Design review of the part built by this model. Coordinates are the model's own, in mm. Face numbers are marked on the shaded views. A direction names the side the tool comes from. Round coordinates to 2 decimals unless told otherwise and drop trailing zeros. One line per question, with ' | ' between items. Start each with the question number.
Item 1: Machinability: for the marked faces 1, 2 and 3, which of the approach directions +Z, -Z, +X, -X, +Y, -Y give a long, thin tool a straight path to every point of the face, cutting with its end or side? Answer none if there is none.
Item 2: For L1, parallel to Y at x = 0, z = 7; L2, parallel to Y at x = 24, z = 4.25; L3, parallel to Y at x = 13.5, z = 6.25, list the stretches that pass through material, from the lowest coordinate up.
Item 3: Insertion check: pin 1 Ø6 at (x, y) = (21.5, -20.5) entering from -Z; pin 2 Ø4 at (x, y) = (20.5, -15) entering from +Z; pin 3 Ø1.2 at (y, z) = (-24.5, 4) entering from -X. Each pin has a flat end and moves straight along its axis. Give the tip position at first contact, or say it passes through.
Item 4: Draft analysis for pull direction X (two halves, no side actions). For the marked faces 4, 5 and 6, state which applies: released by +X, released by -X, zero draft, split by the parting line, or undercut.
Item 5: Add section A-A, the plane z = 1.5. Give the number of separate pieces and of enclosed holes in the cut face, and give its area (3 significant figures).
```python
from build123d import *

# Parameters (mm, degrees)
SKETCH1_R           = 5
SKETCH1_R_2         = 2.55
SKETCH1_R_3         = 1
BOSS_EXTRUDE1_DEPTH = 11
SKETCH2_R           = 19.05
SKETCH2_R_2         = 5
BOSS_EXTRUDE2_DEPTH = 1.6
CUT_EXTRUDE1_DEPTH  = 3
FILLET1_R           = 0.3
CHAMFER1_SIZE       = 0.3
CUT_EXTRUDE2_DEPTH  = 6
CHAMFER2_SIZE       = 0.3
CUT_EXTRUDE3_DEPTH  = 8
SKETCH6_R           = 9
SKETCH6_R_2         = 5
CUT_EXTRUDE4_DEPTH  = 2.6
SKETCH7_R           = 11
SKETCH7_R_2         = 9
CUT_EXTRUDE5_DEPTH  = 1.6
BOSS_EXTRUDE3_START = 3
SKETCH8_R           = 17.5
SKETCH8_R_2         = 11
BOSS_EXTRUDE3_DEPTH = 3
BOSS_EXTRUDE4_START = 7
SKETCH9_R           = 17
SKETCH9_R_2         = 11
BOSS_EXTRUDE4_DEPTH = 7
CHAMFER3_SIZE       = 0.3
CHAMFER4_SIZE       = 0.5
CHAMFER5_SIZE       = 1
CHAMFER5_SIZE2      = 1.732050808


with BuildPart() as part:
    # Sketch1 → Boss-Extrude1 (new body)
    with BuildSketch(Plane.XY):
        with BuildLine():
            Line((-25.2, 28.2), (25.2, 28.2))
            ThreePointArc((25.2, 28.2), (27.321320344, 27.321320344), (28.2, 25.2))
            Line((28.2, 25.2), (28.2, -25.2))
            ThreePointArc((28.2, -25.2), (27.321320344, -27.321320344), (25.2, -28.2))
            Line((25.2, -28.2), (-25.2, -28.2))
            ThreePointArc((-25.2, -28.2), (-27.321320344, -27.321320344), (-28.2, -25.2))
            Line((-28.2, -25.2), (-28.2, 25.2))
            ThreePointArc((-28.2, 25.2), (-27.321320344, 27.321320344), (-25.2, 28.2))
        make_face()
        Circle(SKETCH1_R, mode=Mode.SUBTRACT)
        with Locations((-23.57, 23.57)):
            Circle(SKETCH1_R_2, mode=Mode.SUBTRACT)
        with Locations(Location((23.57, 23.57, 0), (0, 0, 180))):
            Circle(SKETCH1_R_2, mode=Mode.SUBTRACT)
        with Locations((23.57, -23.57)):
            Circle(SKETCH1_R_2, mode=Mode.SUBTRACT)
        with Locations(Location((-23.57, -23.57, 0), (0, 0, 180))):
            Circle(SKETCH1_R_2, mode=Mode.SUBTRACT)
        with Locations((16.2, 25.2)):
            Circle(SKETCH1_R_3, mode=Mode.SUBTRACT)
        with Locations((-25.2, 16.2)):
            Circle(SKETCH1_R_3, mode=Mode.SUBTRACT)
        with Locations((-16.2, -25.2)):
            Circle(SKETCH1_R_3, mode=Mode.SUBTRACT)
        with Locations((25.2, -16.2)):
            Circle(SKETCH1_R_3, mode=Mode.SUBTRACT)
    extrude(amount=BOSS_EXTRUDE1_DEPTH)

    # Sketch2 → Boss-Extrude2 (add)
    with BuildSketch(Plane.XY.offset(11)):
        with Locations(Location((0, 0, 0), (0, 0, 180))):
            Circle(SKETCH2_R)
        Circle(SKETCH2_R_2, mode=Mode.SUBTRACT)
    extrude(amount=BOSS_EXTRUDE2_DEPTH)

    # Sketch3 → Cut-Extrude1 (cut)
    with BuildSketch(Plane.XY.offset(11)):
        with BuildLine():
            Line((13.2, 28.2), (19.2, 28.2))
            Line((19.2, 28.2), (19.2, 25.2))
            ThreePointArc((19.2, 25.2), (16.2, 22.2), (13.2, 25.2))
            Line((13.2, 25.2), (13.2, 28.2))
        make_face()
        with BuildLine():
            Line((-28.2, 13.2), (-28.2, 19.2))
            Line((-28.2, 19.2), (-25.2, 19.2))
            ThreePointArc((-25.2, 19.2), (-22.2, 16.2), (-25.2, 13.2))
            Line((-25.2, 13.2), (-28.2, 13.2))
        make_face()
        with BuildLine():
            Line((28.2, -13.2), (28.2, -19.2))
            Line((28.2, -19.2), (25.2, -19.2))
            ThreePointArc((25.2, -19.2), (22.2, -16.2), (25.2, -13.2))
            Line((25.2, -13.2), (28.2, -13.2))
        make_face()
        with BuildLine():
            Line((-13.2, -28.2), (-13.2, -25.2))
            ThreePointArc((-13.2, -25.2), (-16.2, -22.2), (-19.2, -25.2))
            Line((-19.2, -25.2), (-19.2, -28.2))
            Line((-19.2, -28.2), (-13.2, -28.2))
        make_face()
    extrude(amount=-CUT_EXTRUDE1_DEPTH, mode=Mode.SUBTRACT)

    # Fillet1
    fillet1_edges = [part.edges().sort_by_distance(p)[0] for p in [
        (-27.321320344, 27.321320344, 11),
        (6, -28.2, 11),
        (-28.2, 22.2, 11),
        (-27.321320344, -27.321320344, 11),
        (-22.2, -28.2, 11),
        (27.321320344, -27.321320344, 11),
        (28.2, -22.2, 11),
        (27.321320344, 27.321320344, 11),
        (19.05, 0, 11),
        (19.05, 0, 12.6),
        (22.2, 28.2, 11),
        (-6, 28.2, 11),
        (-28.2, -6, 11),
        (28.2, 6, 11),
    ]]
    fillet(fillet1_edges, radius=FILLET1_R)

    # Chamfer1
    chamfer1_edges = [part.edges().sort_by_distance(p)[0] for p in [
        (28.2, -13.2, 9.35),
        (28.2, -19.2, 9.35),
        (24.2, -16.2, 8),
        (22.2, -16.2, 11),
        (26.55, -19.2, 11),
        (-13.2, -28.2, 9.35),
        (-19.2, -28.2, 9.35),
        (-17.2, -25.2, 8),
        (-16.2, -22.2, 11),
        (-19.2, -26.55, 11),
        (-13.2, -26.55, 11),
        (26.55, -13.2, 11),
        (13.2, 26.55, 11),
        (-26.55, 13.2, 11),
        (-28.112132034, 19.2, 10.912132034),
        (19.2, 28.112132034, 10.912132034),
        (28.112132034, -19.2, 10.912132034),
        (-19.2, -28.112132034, 10.912132034),
        (13.2, 28.112132034, 10.912132034),
        (28.112132034, -13.2, 10.912132034),
        (-13.2, -28.112132034, 10.912132034),
        (-28.112132034, 13.2, 10.912132034),
        (19.2, 28.2, 9.35),
        (13.2, 28.2, 9.35),
        (15.2, 25.2, 8),
        (19.2, 26.55, 11),
        (16.2, 22.2, 11),
        (-28.2, 13.2, 9.35),
        (-28.2, 19.2, 9.35),
        (-26.2, 16.2, 8),
        (-22.2, 16.2, 11),
        (-26.55, 19.2, 11),
    ]]
    chamfer(chamfer1_edges, length=CHAMFER1_SIZE - 0.0001)  # a hair under: the kernel refuses the full size

    # Sketch4 → Cut-Extrude2 (cut)
    with BuildSketch(Plane(origin=(0, 0, 0), x_dir=(-1, 0, 0), z_dir=(0, 0, -1))):
        with BuildLine():
            Line((-23.7, 19.2), (-25.185156579, 19.199963279))
            ThreePointArc((-25.185156579, 19.199963279), (-27.316065894, 18.32656181), (-28.2, 16.2))
            Line((-28.2, 16.2), (-28.2, 25.2))
            ThreePointArc((-28.2, 25.2), (-27.321320344, 27.321320344), (-25.2, 28.2))
            Line((-25.2, 28.2), (-16.2, 28.2))
            ThreePointArc((-16.2, 28.2), (-18.321320344, 27.321320344), (-19.2, 25.2))
            Line((-19.2, 25.2), (-19.2, 23.7))
            ThreePointArc((-19.2, 23.7), (-20.518019485, 20.518019485), (-23.7, 19.2))
        make_face()
        with BuildLine():
            Line((19.2, 23.7), (19.2, 25.2))
            ThreePointArc((19.2, 25.2), (18.321320344, 27.321320344), (16.2, 28.2))
            Line((16.2, 28.2), (25.2, 28.2))
            ThreePointArc((25.2, 28.2), (27.321320344, 27.321320344), (28.2, 25.2))
            Line((28.2, 25.2), (28.2, 16.2))
            ThreePointArc((28.2, 16.2), (27.316065894, 18.32656181), (25.185156579, 19.199963279))
            Line((25.185156579, 19.199963279), (23.7, 19.2))
            ThreePointArc((23.7, 19.2), (20.518019485, 20.518019485), (19.2, 23.7))
        make_face()
        with BuildLine():
            Line((-28.2, -16.2), (-28.2, -25.2))
            ThreePointArc((-28.2, -25.2), (-27.321320344, -27.321320344), (-25.2, -28.2))
            Line((-25.2, -28.2), (-16.2, -28.2))
            ThreePointArc((-16.2, -28.2), (-18.321320344, -27.321320344), (-19.2, -25.2))
            Line((-19.2, -25.2), (-19.2, -23.7))
            ThreePointArc((-19.2, -23.7), (-20.518019485, -20.518019485), (-23.7, -19.2))
            Line((-23.7, -19.2), (-25.185156579, -19.199963279))
            ThreePointArc((-25.185156579, -19.199963279), (-27.316065894, -18.32656181), (-28.2, -16.2))
        make_face()
        with BuildLine():
            Line((28.2, -16.2), (28.2, -25.2))
            ThreePointArc((28.2, -25.2), (27.321320344, -27.321320344), (25.2, -28.2))
            Line((25.2, -28.2), (16.2, -28.2))
            ThreePointArc((16.2, -28.2), (18.321320344, -27.321320344), (19.2, -25.2))
            Line((19.2, -25.2), (19.2, -23.7))
            ThreePointArc((19.2, -23.7), (20.518019485, -20.518019485), (23.7, -19.2))
            Line((23.7, -19.2), (25.185156579, -19.199963279))
            ThreePointArc((25.185156579, -19.199963279), (27.316065894, -18.32656181), (28.2, -16.2))
        make_face()
    extrude(amount=-CUT_EXTRUDE2_DEPTH, mode=Mode.SUBTRACT)

    # Chamfer2
    chamfer2_edges = [part.edges().sort_by_distance(p)[0] for p in [
        (-26.12, 23.57, 11),
        (26.12, 23.57, 11),
        (26.12, 23.57, 6),
        (21.02, -23.57, 11),
        (-26.12, 23.57, 6),
        (21.02, -23.57, 6),
        (-21.02, -23.57, 11),
        (-21.02, -23.57, 6),
    ]]
    chamfer(chamfer2_edges, length=CHAMFER2_SIZE)

    # Sketch5 → Cut-Extrude3 (cut)
    with BuildSketch(Plane(origin=(0, 0, 0), x_dir=(-1, 0, 0), z_dir=(0, 0, -1))):
        Polygon((10.810973978, -26.1), (26.1, -10.810973978), (26.1, 10.810973978), (10.810973978, 26.1), (-10.810973978, 26.1), (-26.1, 10.810973978), (-26.1, -10.810973978), (-10.810973978, -26.1), align=None)
    extrude(amount=-CUT_EXTRUDE3_DEPTH, mode=Mode.SUBTRACT)

    # Sketch6 → Cut-Extrude4 (cut)
    with BuildSketch(Plane(origin=(0, 0, 8), x_dir=(-1, 0, 0), z_dir=(0, 0, -1))):
        Circle(SKETCH6_R)
        Circle(SKETCH6_R_2, mode=Mode.SUBTRACT)
    extrude(amount=-CUT_EXTRUDE4_DEPTH, mode=Mode.SUBTRACT)

    # Sketch7 → Cut-Extrude5 (cut)
    with BuildSketch(Plane(origin=(0, 0, 8), x_dir=(-1, 0, 0), z_dir=(0, 0, -1))):
        Circle(SKETCH7_R)
        Circle(SKETCH7_R_2, mode=Mode.SUBTRACT)
    extrude(amount=-CUT_EXTRUDE5_DEPTH, mode=Mode.SUBTRACT)

    # Sketch8 → Boss-Extrude3 (add)
    with BuildSketch(Plane(origin=(0, 0, 8), x_dir=(-1, 0, 0), z_dir=(0, 0, -1)).offset(BOSS_EXTRUDE3_START)):
        Circle(SKETCH8_R)
        Circle(SKETCH8_R_2, mode=Mode.SUBTRACT)
    extrude(amount=-BOSS_EXTRUDE3_DEPTH)

    # Sketch9 → Boss-Extrude4 (add)
    with BuildSketch(Plane(origin=(0, 0, 5), x_dir=(-1, 0, 0), z_dir=(0, 0, -1)).offset(BOSS_EXTRUDE4_START)):
        Circle(SKETCH9_R)
        Circle(SKETCH9_R_2, mode=Mode.SUBTRACT)
    extrude(amount=-BOSS_EXTRUDE4_DEPTH)

    # Chamfer3
    chamfer3_edges = [part.edges().sort_by_distance(p)[0] for p in [
        (15.2, 25.2, 0),
        (-26.2, 16.2, 0),
        (-17.2, -25.2, 0),
        (0, -26.1, 0),
        (-18.455486989, -18.455486989, 0),
        (-26.1, 0, 0),
        (-18.455486989, 18.455486989, 0),
        (0, 26.1, 0),
        (18.455486989, 18.455486989, 0),
        (26.1, 0, 0),
        (18.455486989, -18.455486989, 0),
        (-5, 0, 10.6),
        (24.2, -16.2, 0),
        (-5, 0, 12.6),
    ]]
    chamfer(chamfer3_edges, length=CHAMFER3_SIZE)

    # Chamfer4
    chamfer4_edges = [part.edges().sort_by_distance(p)[0] for p in [
        (17, 0, -2),
    ]]
    chamfer(chamfer4_edges, length=CHAMFER4_SIZE)

    # Chamfer5
    chamfer5_edges = [part.edges().sort_by_distance(p)[0] for p in [
        (11, 0, -2),
    ]]
    chamfer5_side = [part.faces().sort_by_distance(p)[0] for p in [
        (16.033309524, 0, -2),
    ]]
    chamfer(chamfer5_edges, length=CHAMFER5_SIZE, length2=CHAMFER5_SIZE2, reference=chamfer5_side[0])


solid = part.part
```
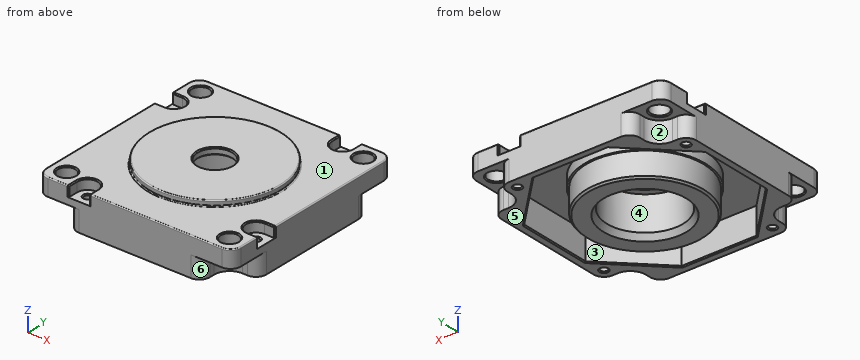
Computed values:
1) face 1: +Z | face 2: -Z, -X, +Y | face 3: -Z
2) L1: y = -28.2 to -26.1, -17.5 to -11, 11 to 17.5, 26.1 to 28.2 | L2: y = -19.2 to -12.91, 12.91 to 19.2 | L3: y = -28.2 to -23.41, -11.14 to 11.14, 23.41 to 28.2
3) pin 1: stops at z = 0 | pin 2: stops at z = 11 | pin 3: stops at x = -19.2
4) face 4: undercut | face 5: zero draft | face 6: released by +X
5) separate pieces: 2 | enclosed holes: 6 | area: 1,120 mm^2
